Geometry: final body of the model. Coordinates: model frame, mm. Face numbers are marked on the shaded views. A direction names the side the tool comes from. Give positions to 0.01 mm unless a question says otherwise; leave off trailing zeros. Order: outer loops, then holes, each group sorted by start corner. A loop starts at its lowest first (then second) coordinate and runs counter-clockwise, first axis right, second up. Notation, with made-up numbers: (3, 44.25) - (48, 44.25) arc R11 ccw to (48, 65.25) - close; hole circle Ø1 at (-25.75, 56). An arc over 180 degrees is marked (long way). One line per item, written item: value.
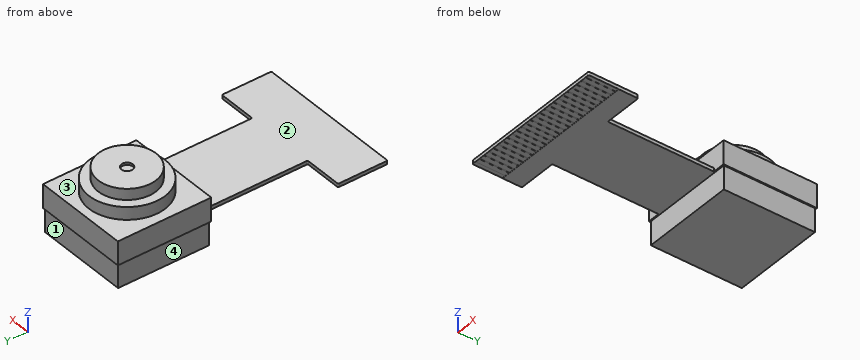
```python
from build123d import *

# Parameters (mm, degrees)
SKETCH1_W           = 8.1
SKETCH1_H           = 7.92
BOSS_EXTRUDE1_DEPTH = 6
SKETCH2_W           = 8.1
SKETCH2_H           = 7.92
SKETCH2_R           = 3.235
CUT_EXTRUDE1_DEPTH  = 2
SKETCH3_R           = 3.235
SKETCH3_R_2         = 2.45
CUT_EXTRUDE2_DEPTH  = 0.93
SKETCH4_R           = 0.48
CUT_EXTRUDE3_DEPTH  = 0.2
SKETCH5_W           = 8.1
SKETCH5_H           = 7.92
SKETCH5_W_2         = 7.9
SKETCH5_H_2         = 7.72
CUT_EXTRUDE4_DEPTH  = 2
BOSS_EXTRUDE2_DEPTH = 0.3
SKETCH7_W           = 12.58
SKETCH7_H           = 2.55
SKETCH7_W_2         = 0.4
SKETCH7_H_2         = 2.54
CUT_EXTRUDE5_DEPTH  = 0.01
FILLET1_START       = 1
FILLET1_DEPTH       = 2
FILLET1_START_2     = 2
FILLET1_2_DEPTH     = 0.3


with BuildPart() as part:
    # Sketch1 → Boss-Extrude1 (new body)
    with BuildSketch(Plane.XY):
        Rectangle(SKETCH1_W, SKETCH1_H)
    extrude(amount=BOSS_EXTRUDE1_DEPTH)

    # Sketch2 → Cut-Extrude1 (cut)
    with BuildSketch(Plane.XY.offset(6)):
        Rectangle(SKETCH2_W, SKETCH2_H)
        Circle(SKETCH2_R, mode=Mode.SUBTRACT)
    extrude(amount=-CUT_EXTRUDE1_DEPTH, mode=Mode.SUBTRACT)

    # Sketch3 → Cut-Extrude2 (cut)
    with BuildSketch(Plane.XY.offset(6)):
        Circle(SKETCH3_R)
        Circle(SKETCH3_R_2, mode=Mode.SUBTRACT)
    extrude(amount=-CUT_EXTRUDE2_DEPTH, mode=Mode.SUBTRACT)

    # Sketch4 → Cut-Extrude3 (cut)
    with BuildSketch(Plane.XY.offset(6)):
        Circle(SKETCH4_R)
    extrude(amount=-CUT_EXTRUDE3_DEPTH, mode=Mode.SUBTRACT)

    # Sketch5 → Cut-Extrude4 (cut)
    with BuildSketch(Plane(origin=(0, 0, 0), x_dir=(-1, 0, 0), z_dir=(0, 0, -1))):
        Rectangle(SKETCH5_W, SKETCH5_H)
        Rectangle(SKETCH5_W_2, SKETCH5_H_2, mode=Mode.SUBTRACT)
    extrude(amount=-CUT_EXTRUDE4_DEPTH, mode=Mode.SUBTRACT)

    # Sketch6 → Boss-Extrude2 (add)
    with BuildSketch(Plane(origin=(0, 0, 2), x_dir=(-1, 0, 0), z_dir=(0, 0, -1))):
        Polygon((-3, -17.16), (3, -17.16), (6.29, -17.16), (6.29, -12.96), (3, -12.96), (3, -3.96), (-3, -3.96), (-3, -12.96), (-6.29, -12.96), (-6.29, -17.16), align=None)
    extrude(amount=-BOSS_EXTRUDE2_DEPTH)

    # Sketch7 → Cut-Extrude5 (cut)
    with BuildSketch(Plane(origin=(0, 0, 2), x_dir=(-1, 0, 0), z_dir=(0, 0, -1))):
        with Locations((0, -15.885)):
            Rectangle(SKETCH7_W, SKETCH7_H)
        with Locations((-5.75, -15.89)):
            Rectangle(SKETCH7_W_2, SKETCH7_H_2, mode=Mode.SUBTRACT)
        with Locations((-5.25, -15.89)):
            Rectangle(SKETCH7_W_2, SKETCH7_H_2, mode=Mode.SUBTRACT)
        with Locations((-4.75, -15.89)):
            Rectangle(SKETCH7_W_2, SKETCH7_H_2, mode=Mode.SUBTRACT)
        with Locations((-4.25, -15.89)):
            Rectangle(SKETCH7_W_2, SKETCH7_H_2, mode=Mode.SUBTRACT)
        with Locations((-3.75, -15.89)):
            Rectangle(SKETCH7_W_2, SKETCH7_H_2, mode=Mode.SUBTRACT)
        with Locations((-3.25, -15.89)):
            Rectangle(SKETCH7_W_2, SKETCH7_H_2, mode=Mode.SUBTRACT)
        with Locations((-2.75, -15.89)):
            Rectangle(SKETCH7_W_2, SKETCH7_H_2, mode=Mode.SUBTRACT)
        with Locations((-2.25, -15.89)):
            Rectangle(SKETCH7_W_2, SKETCH7_H_2, mode=Mode.SUBTRACT)
        with Locations((-1.75, -15.89)):
            Rectangle(SKETCH7_W_2, SKETCH7_H_2, mode=Mode.SUBTRACT)
        with Locations((-1.25, -15.89)):
            Rectangle(SKETCH7_W_2, SKETCH7_H_2, mode=Mode.SUBTRACT)
        with Locations((-0.75, -15.89)):
            Rectangle(SKETCH7_W_2, SKETCH7_H_2, mode=Mode.SUBTRACT)
        with Locations((-0.25, -15.89)):
            Rectangle(SKETCH7_W_2, SKETCH7_H_2, mode=Mode.SUBTRACT)
        with Locations((0.25, -15.89)):
            Rectangle(SKETCH7_W_2, SKETCH7_H_2, mode=Mode.SUBTRACT)
        with Locations((0.75, -15.89)):
            Rectangle(SKETCH7_W_2, SKETCH7_H_2, mode=Mode.SUBTRACT)
        with Locations((1.25, -15.89)):
            Rectangle(SKETCH7_W_2, SKETCH7_H_2, mode=Mode.SUBTRACT)
        with Locations((1.75, -15.89)):
            Rectangle(SKETCH7_W_2, SKETCH7_H_2, mode=Mode.SUBTRACT)
        with Locations((2.25, -15.89)):
            Rectangle(SKETCH7_W_2, SKETCH7_H_2, mode=Mode.SUBTRACT)
        with Locations((2.75, -15.89)):
            Rectangle(SKETCH7_W_2, SKETCH7_H_2, mode=Mode.SUBTRACT)
        with Locations((3.25, -15.89)):
            Rectangle(SKETCH7_W_2, SKETCH7_H_2, mode=Mode.SUBTRACT)
        with Locations((3.75, -15.89)):
            Rectangle(SKETCH7_W_2, SKETCH7_H_2, mode=Mode.SUBTRACT)
        with Locations((4.25, -15.89)):
            Rectangle(SKETCH7_W_2, SKETCH7_H_2, mode=Mode.SUBTRACT)
        with Locations((4.75, -15.89)):
            Rectangle(SKETCH7_W_2, SKETCH7_H_2, mode=Mode.SUBTRACT)
        with Locations((5.25, -15.89)):
            Rectangle(SKETCH7_W_2, SKETCH7_H_2, mode=Mode.SUBTRACT)
        with Locations((5.75, -15.89)):
            Rectangle(SKETCH7_W_2, SKETCH7_H_2, mode=Mode.SUBTRACT)
    extrude(amount=-CUT_EXTRUDE5_DEPTH, mode=Mode.SUBTRACT)

    # Fillet1: read off the stored shape, not the designer's step
    # Fillet1 outline → Fillet1 (cut)
    with BuildSketch(Plane.XY.offset(FILLET1_START)):
        with BuildLine():
            ThreePointArc((6.19, -12.96), (6.260710678, -12.989289322), (6.29, -13.06))
            Line((6.29, -13.06), (6.29, -12.96))
            Line((6.29, -12.96), (6.19, -12.96))
        make_face()
        with BuildLine():
            ThreePointArc((6.29, -17.06), (6.260710678, -17.130710678), (6.19, -17.16))
            Line((6.19, -17.16), (6.29, -17.16))
            Line((6.29, -17.16), (6.29, -17.06))
        make_face()
        with BuildLine():
            Line((-6.29, -12.96), (-6.29, -13.06))
            ThreePointArc((-6.29, -13.06), (-6.260710678, -12.989289322), (-6.19, -12.96))
            Line((-6.19, -12.96), (-6.29, -12.96))
        make_face()
        with BuildLine():
            ThreePointArc((-6.19, -17.16), (-6.260710678, -17.130710678), (-6.29, -17.06))
            Line((-6.29, -17.06), (-6.29, -17.16))
            Line((-6.29, -17.16), (-6.19, -17.16))
        make_face()
    extrude(amount=FILLET1_DEPTH, mode=Mode.SUBTRACT)

    # Fillet1 2 outline → Fillet1 2 (add)
    with BuildSketch(Plane.XY.offset(FILLET1_START_2)):
        with BuildLine():
            Line((3, -12.96), (3.1, -12.96))
            ThreePointArc((3.1, -12.96), (3.029289322, -12.930710678), (3, -12.86))
            Line((3, -12.86), (3, -12.96))
        make_face()
        with BuildLine():
            ThreePointArc((-3, -12.86), (-3.029289322, -12.930710678), (-3.1, -12.96))
            Line((-3.1, -12.96), (-3, -12.96))
            Line((-3, -12.96), (-3, -12.86))
        make_face()
    extrude(amount=FILLET1_2_DEPTH)


solid = part.part
```
1) Section B-B, the plane z = 1.15. Return loops of the section in (x, y), then the cut area to 3 significant figures.
Answers below:
outline: (-3.95, -3.86) - (3.95, -3.86) - (3.95, 3.86) - (-3.95, 3.86) - close
area: 61.0 mm^2
2) Set-up query: the marked faces 1, 2, 3 and 4. Return all of +Z, -Z, +X, -X, +Y, -Y with unobstructed straight access to the full face (end or side cutting, diameter ignored); none if empty.
Answers below:
face 1: -Z, +X, -X, +Y
face 2: +Z, +X, -X, -Y
face 3: +Z
face 4: -Z, -X, +Y, -Y
3) Section D-D, the plane z = 4.6. Return loops of the section in (x, y) (3 decimals), then the cut area to 3 significant figures.
Answers below:
outline: circle Ø6.47 at (0, 0)
area: 32.9 mm^2
4) Section A-A, the plane y = 0. Return loops of the section in (x, z) (3 decimals), then the cut area to 3 significant figures.
Answers below:
outline: (-4.05, 2) - (-3.95, 2) - (-3.95, 0) - (3.95, 0) - (3.95, 2) - (4.05, 2) - (4.05, 4) - (3.235, 4) - (3.235, 5.07) - (2.45, 5.07) - (2.45, 6) - (0.48, 6) - (0.48, 5.8) - (-0.48, 5.8) - (-0.48, 6) - (-2.45, 6) - (-2.45, 5.07) - (-3.235, 5.07) - (-3.235, 4) - (-4.05, 4) - close
area: 43.3 mm^2
5) First-contact query: pin 1 (5 mm diameter, centred on x = -1.5, y = -8.5, fed in from -Z); pin 2 (2 mm diameter, centred on x = 1, y = -12, fed in from +Z). Flat tips, straight axial feed; report the tip coordinate or a pass-through.
Answers below:
pin 1: z = 2
pin 2: z = 2.3
6) Section C-C, the plane y = -3. Return loops of the section in (x, z).
Answers below:
outline: (-4.05, 2) - (-3.95, 2) - (-3.95, 0) - (3.95, 0) - (3.95, 2) - (4.05, 2) - (4.05, 4) - (1.21, 4) - (1.21, 5.07) - (-1.21, 5.07) - (-1.21, 4) - (-4.05, 4) - close
7) Material intervals for line 1 along Y through (x, z) = (0, 5.95); line 2 along Y through (x, z) = (0.25, 2.4); line 3 along Z through (x, y) = (-0.75, -12.5), sorted ascending.
Answers below:
line 1: -2.45 to -0.48, 0.48 to 2.45
line 2: -3.96 to 3.96
line 3: 2 to 2.3
